Input: dimensioned drawing with shaded views. Units: mm. Origin: part minimum x, y, z. A direction names the side the tool comes from. Give positions to 0.01 mm unless a question says otherwise; leave off trailing zeros. Write each loop counter-clockwise with the first axis right and the second up, starting at its lowest first coordinate (ties: lowest second). Pieces come first, ordered by that corner, then holes. Notation, with made-up numbers: M 70,2.5 L 83,2.5 A12 cw 83,12.5 Z; hole C -14,44 d11. An arc over 180 degrees is marked long. Use CSV: the item, a comma, the result in double quotes. Start each with the question number.
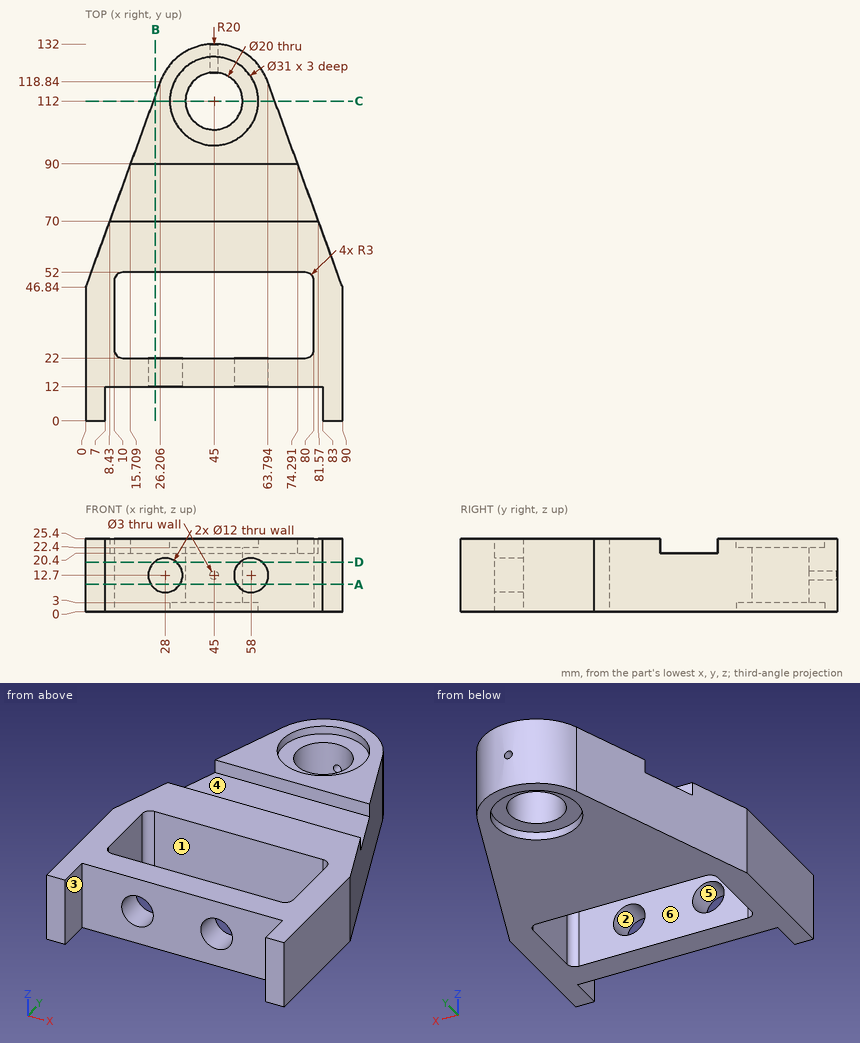
Q1. Section B-B, the plane x = 24.5. Return the cut outline in (y, z), and give its area (3 significant figures).
Q2. Section C-C, the plane y = 112. Return the cut outline in (x, z).
Q3. Section D-D, the plane z = 17.25. Return the cut outline in (x, y), and give its area (3 significant figures).
Q4. Pull-direction query (Z, two-part tool) for the marked faces 4, 5 and 6; classes: released by +Z, released by -Z, zero draft, split by the parting line, or undercut.
Q5. First-contact query: pin 1 Ø7.5 at (x, z) = (30.5, 18.5) entering from +Y (1 decimal); pin 2 Ø3 at (y, z) = (68.5, 17) entering from -X; pin 3 Ø1 at (x, z) = (47.5, 9.5) entering from -Y; pin 4 Ø16 at (x, y) = (45, 112) entering from -Z (3 decimals). Flat tips, straight axial feed; report the tip coordinate or a pass-through.
Q6. Set-up query: the marked faces 1, 2 and 3. Return all of +Z, -Z, +X, -X, +Y, -Y with unobstructed straight access to the full face (end or side cutting, diameter ignored); none if empty.
Q7. Material intervals for L1, parallel to Z at x = 45, y = 125.75; L2, parallel to X at y = 9, z = 4.5; L3, parallel to Y at x = 45, z = 11.75, sorted ascending. Write a range as [from, to].
Q8. Section A-A, the plane z = 9.5. Return the cut outline in (x, y) (1 decimal), and give its area (3 significant figures).
Check result:
1,outline,"M 12,0 L 22,0 L 22,7.83 L 12,7.83 Z; M 12,17.57 L 22,17.57 L 22,25.4 L 12,25.4 Z; M 52,0 L 114.15,0 L 114.15,25.4 L 90,25.4 L 90,20.4 L 70,20.4 L 70,25.4 L 52,25.4 Z"
1,area,"1,640 mm²"
2,outline,"M 23.72,0 L 29.5,0 L 29.5,3 L 35,3 L 35,22.4 L 29.5,22.4 L 29.5,25.4 L 23.72,25.4 Z; M 55,3 L 60.5,3 L 60.5,0 L 66.28,0 L 66.28,25.4 L 60.5,25.4 L 60.5,22.4 L 55,22.4 Z"
3,outline,"M 0,0 L 7,0 L 7,12 L 24.09,12 L 24.09,22 L 13,22 A3 cw 10,25 L 10,49 A3 cw 13,52 L 77,52 A3 cw 80,49 L 80,25 A3 cw 77,22 L 61.91,22 L 61.91,12 L 83,12 L 83,0 L 90,0 L 90,46.84 L 63.79,118.84 A20 ccw 26.21,118.84 L 0,46.84 Z; M 31.91,12 L 54.09,12 L 54.09,22 L 31.91,22 Z; hole C 45,112 d20"
3,area,"5,690 mm²"
4,face 4,"released by +Z"
4,face 5,"undercut"
4,face 6,"zero draft"
5,pin 1,"stops at y = 128.9"
5,pin 2,"stops at x = 7.34"
5,pin 3,"stops at y = 12"
5,pin 4,"passes through"
6,face 1,"+Z, -Z"
6,face 2,"-Y"
6,face 3,"+Z, -Z, -Y"
7,L1,"z = [3, 11.2], [14.2, 22.4]"
7,L2,"x = [0, 7], [83, 90]"
7,L3,"y = [12, 22], [52, 102]"
8,outline,"M 0,0 L 7,0 L 7,12 L 22.9,12 L 22.9,22 L 13,22 A3 cw 10,25 L 10,49 A3 cw 13,52 L 77,52 A3 cw 80,49 L 80,25 A3 cw 77,22 L 63.1,22 L 63.1,12 L 83,12 L 83,0 L 90,0 L 90,46.8 L 63.8,118.8 A20 ccw 26.2,118.8 L 0,46.8 Z; M 33.1,12 L 52.9,12 L 52.9,22 L 33.1,22 Z; hole C 45,112 d20"
8,area,"5,650 mm²"
